Input: part model. Units: mm. Frame: model coordinates. A direction names the side the tool comes from. Round coordinates to 2 decimals unless told otherwise and drop trailing zeros. Order: outer loops, then holes, each group sorted by start corner. A loop starts at its lowest first (then second) coordinate and runs counter-clockwise, first axis right, second up.
Item 1: Cut plane A-A on z = 1.25. Output: boundary loops of the cut face in (x, y).
Item 2: Line query: L1, parallel to Y at x = 10, z = 3.35; L2, parallel to Z at x = 7, y = 18.5; L3, parallel to Y at x = 14.25, z = 6. Output: solid intervals per line, ascending.
Item 3: Cut plane C-C on y = 23.75. Output: boundary loops of the cut face in (x, z).
Item 4: Cut plane B-B on x = 10. Output: boundary loops of the cut face in (y, z).
Item 5: First-contact query: pin 1 (5 mm diameter, centred on x = 3.5, z = 4, fed in from +Y); pin 2 (2 mm diameter, centred on x = 6.5, y = 23, fed in from +Z); pin 3 (4.5 mm diameter, centred on x = 7, z = 7.5, fed in from +Y). Flat tips, straight axial feed; report the tip coordinate or a pass-through.
Item 6: Cut plane D-D on z = 3.6. Output: boundary loops of the cut face in (x, y).
Item 7: Reachability of faces 1 (the flat face through (10, 4, 8.4)), 2 (the flat face through (10, 16, 4.2)), 3 (the flat face through (15, 5.5, 3.6)) from +Z, -Z, +X, -X, +Y, -Y: full face, straight path, thin tool, end or side. Return the list, or none.
Item 8: Mould query, pull axis Z, two halves, no side actions, for faces 4 (the flat face through (10, 12, 0)), 5 (the cylindrical face through (14.5, 2.7, 3.6)), 6 (the flat face through (20, 3, 4)). Classes: released by +Z, released by -Z, zero draft, split by the parting line, or undercut.
Autodesk Inventor part; units mm, degrees
ref_plane "YZ Plane" through (0, 0, 0) normal (1, 0, 0) x (0, 1, 0)
ref_plane "XZ Plane" through (0, 0, 0) normal (0, 1, 0) x (-1, 0, 0)
ref_plane "XY Plane" through (0, 0, 0) normal (0, 0, 1) x (1, 0, 0)
sketch "Sketch1" plane through (0, 0, 0) normal (0, 0, 1) x (1, 0, 0)
  circle A0 centre (10, 24.7) radius 1.6
  line L0 (0, 0) -> (20.0001, 0)
  line L1 (0, 0) -> (0, 7)
  line L2 (20.0001, 0) -> (20.0001, 6.9998)
  line L3 (0, 7) -> (4.9176, 25.3526)
  line L4 (0, 7) -> (19, 7) construction
  line L5 (20.0001, 6.9998) -> (15.0825, 25.3524)
  line L6 (20.0001, 6.9998) -> (39.0001, 6.9998) construction
  arc A1 (15.0825, 25.3524) -> (4.9176, 25.3526) centre (10, 23.9906) ccw
  dimension "d17" = 7
  dimension "d18" = 6.9998
  dimension "d19" = 24.7
  dimension "d23" = 90
  dimension "d24" = 90
  dimension "d25" = 10
  dimension "d26" = 19
  dimension "d27" = 75
  dimension "d28" = 19
  dimension "d29" = 105
  dimension "d30" = 10
sketch "Sketch3" plane through (0, 0, 0) normal (0, 0, 1) x (1, 0, 0)
  point P0 (0, 0)
extrude "Extrusion1" add sketch "Sketch1" along normal blind 4.2
sketch "Sketch4" plane through (0, 0, 4.2) normal (0, 0, 1) x (1, 0, 0)
  line L0 (0, 7) -> (0, 0)
  line L1 (20.0001, 0) -> (20.0001, 6.9998)
  line L2 (0, 0) -> (20.0001, 0)
  line L3 (20.0001, 0) -> (20.0001, 6.9998)
  line L4 (3.884, 22.9404) -> (-0.0481, 7.0119)
  line L5 (20.0001, 6.9998) -> (0, 6.9998)
  line L6 (0, 7) -> (0, 0)
extrude "Extrusion2" add sketch "Sketch4" along normal blind 4.2
sketch "Sketch5" plane through (0, 0, 0) normal (0, -1, 0) x (1, 0, 0)
  circle A0 centre (5, 3.6) radius 0.5
  circle A1 centre (15, 3.6) radius 0.5
  line L0 (0, 0) -> (20.0001, 0)
  line L1 (0, 8.4) -> (20.0001, 8.4)
  dimension "d13" = 1
  dimension "d14" = 1
  dimension "d33" = 4.8
  dimension "d34" = 4.8
extrude "Extrusion3" cut sketch "Sketch5" against normal blind 5.5
properties part number "upper_deck_shaft_mount_printing"
From the geometry:
1. outline: (0, 0) - (20, 0) - (20, 7) - (15.08, 25.35) arc R5.26 ccw to (4.92, 25.35) - (0, 7) - close; hole circle Ø3.2 at (10, 24.7)
2. L1: y = 0 to 23.1, 26.3 to 29.25
2. L2: z = 0 to 4.2
2. L3: y = 0 to 7
3. outline: (4.49, 0) - (8.71, 0) - (8.71, 4.2) - (4.49, 4.2) - close; (11.29, 0) - (15.51, 0) - (15.51, 4.2) - (11.29, 4.2) - close
4. outline: (0, 0) - (23.1, 0) - (23.1, 4.2) - (7, 4.2) - (7, 8.4) - (0, 8.4) - close; (26.3, 0) - (29.25, 0) - (29.25, 4.2) - (26.3, 4.2) - close
5. pin 1: stops at y = 27.41
5. pin 2: stops at z = 4.2
5. pin 3: stops at y = 7
6. outline: (0, 0) - (4.5, 0) - (4.5, 5.5) - (5.5, 5.5) - (5.5, 0) - (14.5, 0) - (14.5, 5.5) - (15.5, 5.5) - (15.5, 0) - (20, 0) - (20, 7) - (15.08, 25.35) arc R5.26 ccw to (4.92, 25.35) - (0, 7) - close; hole circle Ø3.2 at (10, 24.7)
7. face 1: +Z, +X, -X, +Y, -Y
7. face 2: +Z, +X, -X, +Y
7. face 3: -Y
8. face 4: released by -Z
8. face 5: undercut
8. face 6: zero draft
